Input: part model. Units: mm. Frame: model coordinates. A direction names the side the tool comes from. Coordinates: 2 decimals unless noted, no trailing zeros. Loops run counter-clockwise (first coordinate to the right, second up) from the corner with the lowest first, then second, coordinate; pieces in that order, holes last. Notation, with made-up numbers: (3.5, -22) -> (51.5, -22) arc R35 ccw to (51.5, 10) -> close; hole circle Ø8 at (47.5, 34). An arc over 180 degrees is marked (long way). Answer as a JSON object with one key per item and string values.
from build123d import *

# Parameters (mm, degrees)
SKETCH2_R               = 5
BOSS_EXTRUDE1_DEPTH     = 4
CUT_EXTRUDE1_DEPTH      = 19.172781887
CUT_EXTRUDE1_DEPTH_BACK = 19.172781887
SKETCH3_R               = 3


with BuildPart() as part:
    # Sketch1 → Revolve1 (revolve)
    with BuildSketch(Plane.XY, mode=Mode.PRIVATE) as revolve1_sk:
        with BuildLine():
            Line((1, 0), (3, 0))
            Line((3, 0), (3, 7.5))
            Line((3, 7.5), (0, 7.5))
            Line((0, 7.5), (0, 1))
            ThreePointArc((0, 1), (0.292893219, 0.292893219), (1, 0))
        make_face()
    revolve(revolve1_sk.sketch.rotate(Axis((0, 7.5, 0), (1, 0, 0)), 270), axis=Axis((0, 7.5, 0), (1, 0, 0)))

    # Sketch2 → Boss-Extrude1 (add)
    with BuildSketch(Plane(origin=(3, 0, 0), x_dir=(0, 0, -1), z_dir=(1, 0, 0))):
        with Locations((0, 7.5)):
            Circle(SKETCH2_R)
    extrude(amount=BOSS_EXTRUDE1_DEPTH)

    # Sketch3 → Cut-Extrude1 (cut, two sides: drawn at the far end of the back side and taken through both)
    with BuildSketch(Plane.ZY.offset(-CUT_EXTRUDE1_DEPTH_BACK)):
        with Locations((0, 7.5)):
            Circle(SKETCH3_R)
    extrude(amount=CUT_EXTRUDE1_DEPTH + CUT_EXTRUDE1_DEPTH_BACK, mode=Mode.SUBTRACT)


solid = part.part
1. Access query for faces 1 (the face through (3, 12.4, 1.6)), 2 (the face through (2.014, 0.064, -0.976)). Directions: +Z, -Z, +X, -X, +Y, -Y. A direction counts if a zero-diameter tool reaches every point of the face in a straight line with its end or side. Return the directions, or none.
Reply:
{"face 1": "+X", "face 2": "+X, -X"}
2. Section query C-C (x = 6). Return loops of the section in (y, z).
Reply:
{"outline": "circle Ø10 at (7.5, 0); hole circle Ø6 at (7.5, 0)"}
3. Mould query, pull axis Y, two halves, no side actions, for faces 3 (the face through (0, 9, -3)), 4 (the face through (3.5, 7.6, -3)), 5 (the face through (4.972, 12.457, 0.651)). Classes: pulls with the +Y half, pulls with the -Y half, needs draft (parallel to the pull), parting line crosses it, or undercut.
Reply:
{"face 3": "needs draft", "face 4": "undercut", "face 5": "parting line crosses it"}
4. Line query: line 1 along Y through (x, z) = (4.75, 0); line 2 along Y through (x, z) = (2, 0); line 3 along Z through (x, y) = (1.25, 8.5). Output: solid intervals per line, ascending.
Reply:
{"line 1": "y = 2.5 to 4.5, 10.5 to 12.5", "line 2": "y = 0 to 4.5, 10.5 to 15", "line 3": "z = -7.43 to -2.83, 2.83 to 7.43"}
5. Section query D-D (x = 2). Return loops of the section in (y, z), plus the area to 3 significant figures.
Reply:
{"outline": "circle Ø15 at (7.5, 0); hole circle Ø6 at (7.5, 0)", "area": "148 mm2"}
6. Section query A-A (y = 7.5). Return loops of the section in (x, z).
Reply:
{"outline": "(0, -6.5) arc R1 ccw to (1, -7.5) -> (3, -7.5) -> (3, -5) -> (7, -5) -> (7, -3) -> (0, -3) -> close; (0, 3) -> (7, 3) -> (7, 5) -> (3, 5) -> (3, 7.5) -> (1, 7.5) arc R1 ccw to (0, 6.5) -> close"}
7. Pin query (flat end, axial travel): P1, Ø6, axis at y = 7, z = -2, coming from the -X side. Return the tip coordinate at first contact, or that it passes through.
Reply:
{"P1": "stops at x = 0"}
8. Section query B-B (z = 0). Return loops of the section in (x, y).
Reply:
{"outline": "(0, 1) arc R1 ccw to (1, 0) -> (3, 0) -> (3, 2.5) -> (7, 2.5) -> (7, 4.5) -> (0, 4.5) -> close; (0, 10.5) -> (7, 10.5) -> (7, 12.5) -> (3, 12.5) -> (3, 15) -> (1, 15) arc R1 ccw to (0, 14) -> close"}
